from build123d import *

# Parameters (mm, degrees)
BOSS_EXTRUDE1_DEPTH                            = 60
CUT_EXTRUDE1_DEPTH                             = 114.247516529
CBORE_FOR_4_SOCKET_HEAD_CAP_SCREW1_D           = 3.2639
CBORE_FOR_4_SOCKET_HEAD_CAP_SCREW1_CBORE_D     = 5.55752
CBORE_FOR_4_SOCKET_HEAD_CAP_SCREW1_CBORE_DEPTH = 2.8448
CUT_EXTRUDE5_REACH                             = 115.248
CUT_EXTRUDE6_DEPTH                             = 2.84
M3_TAPPED_HOLE1_D                              = 2.5
M3_TAPPED_HOLE1_DEPTH                          = 8.5
M3_TAPPED_HOLE1_TIP                            = 0.751075774
M5_TAPPED_HOLE1_D                              = 4.2
SKETCH11_R                                     = 5
CUT_EXTRUDE2_DEPTH                             = 114.247516529
M4_TAPPED_HOLE1_D                              = 3.3
M4_TAPPED_HOLE1_DEPTH                          = 6
M4_TAPPED_HOLE1_CSINK_D                        = 4.5
M4_TAPPED_HOLE1_CSINK_ANGLE                    = 90
M5_TAPPED_HOLE2_D                              = 4.2
M5_TAPPED_HOLE2_DEPTH                          = 6
M5_TAPPED_HOLE2_CSINK_D                        = 5.05
M5_TAPPED_HOLE2_CSINK_ANGLE                    = 90
SKETCH16_R                                     = 10
CUT_EXTRUDE4_DEPTH                             = 30
M3_TAPPED_HOLE2_AT_2_COUNT                     = 2
M3_TAPPED_HOLE2_AT_2_PITCH                     = 20


with BuildPart() as part:
    # Sketch1 → Boss-Extrude1 (new body)
    with BuildSketch(Plane.XY):
        Polygon((0, 0), (6, 0), (6, 54), (69, 54), (69, 40), (75, 40), (75, 60), (0, 60), align=None)
    extrude(amount=BOSS_EXTRUDE1_DEPTH)

    # Sketch2 → Cut-Extrude1 (cut, through all)
    with BuildSketch(Plane(origin=(0, 60, 0), x_dir=(1, 0, 0), z_dir=(0, 1, 0))):
        with BuildLine():
            Line((40, -18.5), (50, -18.5))
            ThreePointArc((50, -18.5), (61.5, -30), (50, -41.5))
            Line((50, -41.5), (40, -41.5))
            ThreePointArc((40, -41.5), (28.5, -30), (40, -18.5))
        make_face()
    extrude(amount=-CUT_EXTRUDE1_DEPTH, mode=Mode.SUBTRACT)

    # CBORE for #4 Socket Head Cap Screw1 (through all)
    with Locations(Plane(origin=(0, 60, 0), x_dir=(-1, 0, 0), z_dir=(0, 1, 0))):
        with Locations((-24.5, 45.5), (-55.5, 45.5), (-24.5, 14.5), (-55.5, 14.5)):
            CounterBoreHole(CBORE_FOR_4_SOCKET_HEAD_CAP_SCREW1_D / 2, CBORE_FOR_4_SOCKET_HEAD_CAP_SCREW1_CBORE_D / 2, CBORE_FOR_4_SOCKET_HEAD_CAP_SCREW1_CBORE_DEPTH)

    # Sketch24 → Cut-Extrude5 (cut, up to next)
    with BuildSketch(Plane(origin=(0, 60, 0), x_dir=(1, 0, 0), z_dir=(0, 1, 0)), mode=Mode.PRIVATE) as cut_extrude5_sk1:
        with BuildLine():
            Line((24.5, -12.86805), (34.5, -12.86805))
            ThreePointArc((34.5, -12.86805), (36.13195, -14.5), (34.5, -16.13195))
            Line((34.5, -16.13195), (24.5, -16.13195))
            ThreePointArc((24.5, -16.13195), (22.86805, -14.5), (24.5, -12.86805))
        make_face()
    cut_extrude5_tool1 = extrude(cut_extrude5_sk1.sketch, amount=-CUT_EXTRUDE5_REACH, mode=Mode.PRIVATE) & part.part
    # Sketch24 → Cut-Extrude5 (cut, up to next)
    with BuildSketch(Plane(origin=(0, 60, 0), x_dir=(1, 0, 0), z_dir=(0, 1, 0)), mode=Mode.PRIVATE) as cut_extrude5_sk2:
        with BuildLine():
            Line((55.5, -12.86805), (65.5, -12.86805))
            ThreePointArc((65.5, -12.86805), (67.13195, -14.5), (65.5, -16.13195))
            Line((65.5, -16.13195), (55.5, -16.13195))
            ThreePointArc((55.5, -16.13195), (53.86805, -14.5), (55.5, -12.86805))
        make_face()
    cut_extrude5_tool2 = extrude(cut_extrude5_sk2.sketch, amount=-CUT_EXTRUDE5_REACH, mode=Mode.PRIVATE) & part.part
    # Sketch24 → Cut-Extrude5 (cut, up to next)
    with BuildSketch(Plane(origin=(0, 60, 0), x_dir=(1, 0, 0), z_dir=(0, 1, 0)), mode=Mode.PRIVATE) as cut_extrude5_sk3:
        with BuildLine():
            Line((24.5, -43.911016089), (34.5, -43.911016089))
            ThreePointArc((34.5, -43.911016089), (36.13195, -45.542966089), (34.5, -47.174916089))
            Line((34.5, -47.174916089), (24.5, -47.174916089))
            ThreePointArc((24.5, -47.174916089), (22.86805, -45.542966089), (24.5, -43.911016089))
        make_face()
    cut_extrude5_tool3 = extrude(cut_extrude5_sk3.sketch, amount=-CUT_EXTRUDE5_REACH, mode=Mode.PRIVATE) & part.part
    # Sketch24 → Cut-Extrude5 (cut, up to next)
    with BuildSketch(Plane(origin=(0, 60, 0), x_dir=(1, 0, 0), z_dir=(0, 1, 0)), mode=Mode.PRIVATE) as cut_extrude5_sk4:
        with BuildLine():
            Line((55.5, -43.911016089), (65.5, -43.911016089))
            ThreePointArc((65.5, -43.911016089), (67.13195, -45.542966089), (65.5, -47.174916089))
            Line((65.5, -47.174916089), (55.5, -47.174916089))
            ThreePointArc((55.5, -47.174916089), (53.86805, -45.542966089), (55.5, -43.911016089))
        make_face()
    cut_extrude5_tool4 = extrude(cut_extrude5_sk4.sketch, amount=-CUT_EXTRUDE5_REACH, mode=Mode.PRIVATE) & part.part
    add(cut_extrude5_tool1.solids().sort_by_distance((29.5, 60, 14.5))[0], mode=Mode.SUBTRACT)
    add(cut_extrude5_tool2.solids().sort_by_distance((60.5, 60, 14.5))[0], mode=Mode.SUBTRACT)
    add(cut_extrude5_tool3.solids().sort_by_distance((29.5, 60, 45.542966))[0], mode=Mode.SUBTRACT)
    add(cut_extrude5_tool4.solids().sort_by_distance((60.5, 60, 45.542966))[0], mode=Mode.SUBTRACT)

    # Sketch25 → Cut-Extrude6 (cut)
    with BuildSketch(Plane(origin=(0, 60, 0), x_dir=(1, 0, 0), z_dir=(0, 1, 0))):
        with BuildLine():
            Line((24.5, -11.72124), (34.5, -11.72124))
            ThreePointArc((34.5, -11.72124), (37.27876, -14.5), (34.5, -17.27876))
            Line((34.5, -17.27876), (24.5, -17.27876))
            ThreePointArc((24.5, -17.27876), (21.72124, -14.5), (24.5, -11.72124))
        make_face()
        with BuildLine():
            Line((55.499999686, -11.73110797), (65.499999686, -11.73110797))
            ThreePointArc((65.499999686, -11.73110797), (68.278759686, -14.50986797), (65.499999686, -17.28862797))
            Line((65.499999686, -17.28862797), (55.499999686, -17.28862797))
            ThreePointArc((55.499999686, -17.28862797), (52.721239686, -14.50986797), (55.499999686, -11.73110797))
        make_face()
        with BuildLine():
            Line((24.5, -42.822083884), (34.5, -42.822083884))
            ThreePointArc((34.5, -42.822083884), (37.27876, -45.600843884), (34.5, -48.379603884))
            Line((34.5, -48.379603884), (24.5, -48.379603884))
            ThreePointArc((24.5, -48.379603884), (21.72124, -45.600843884), (24.5, -42.822083884))
        make_face()
        with BuildLine():
            Line((55.499999686, -42.831951854), (65.499999686, -42.831951854))
            ThreePointArc((65.499999686, -42.831951854), (68.278759686, -45.610711854), (65.499999686, -48.389471854))
            Line((65.499999686, -48.389471854), (55.499999686, -48.389471854))
            ThreePointArc((55.499999686, -48.389471854), (52.721239686, -45.610711854), (55.499999686, -42.831951854))
        make_face()
    extrude(amount=-CUT_EXTRUDE6_DEPTH, mode=Mode.SUBTRACT)

    # M3 Tapped Hole1
    with Locations(Plane(origin=(0, 60, 0), x_dir=(-1, 0, 0), z_dir=(0, 1, 0))):
        with Locations((-12, 55), (-72, 55), (-12, 5), (-72, 5)):
            Hole(M3_TAPPED_HOLE1_D / 2, depth=M3_TAPPED_HOLE1_DEPTH)
            with Locations((0, 0, -(M3_TAPPED_HOLE1_DEPTH + M3_TAPPED_HOLE1_TIP / 2))):  # 118° drill point
                Cone(0, M3_TAPPED_HOLE1_D / 2, M3_TAPPED_HOLE1_TIP, mode=Mode.SUBTRACT)

    # M5 Tapped Hole1 (through all)
    with Locations(Plane(origin=(0, 60, 0), x_dir=(-1, 0, 0), z_dir=(0, 1, 0))):
        with Locations((-44, 12), (-44, 48)):
            Hole(M5_TAPPED_HOLE1_D / 2)

    # Sketch11 → Cut-Extrude2 (cut, through all)
    with BuildSketch(Plane(origin=(0, 60, 0), x_dir=(1, 0, 0), z_dir=(0, 1, 0))):
        with Locations(Location((12, -30, 0), (0, 0, 270))):
            Circle(SKETCH11_R)
    extrude(amount=-CUT_EXTRUDE2_DEPTH, mode=Mode.SUBTRACT)

    # M4 Tapped Hole1
    with Locations(Plane.ZY):
        with Locations((11, 46), (11, 16), (49, 46), (49, 16)):
            CounterSinkHole(M4_TAPPED_HOLE1_D / 2, M4_TAPPED_HOLE1_CSINK_D / 2, depth=M4_TAPPED_HOLE1_DEPTH, counter_sink_angle=M4_TAPPED_HOLE1_CSINK_ANGLE)

    # M5 Tapped Hole2
    with Locations(Plane(origin=(75, 0, 0), x_dir=(0, 0, -1), z_dir=(1, 0, 0))):
        with Locations((-30, 50)):
            CounterSinkHole(M5_TAPPED_HOLE2_D / 2, M5_TAPPED_HOLE2_CSINK_D / 2, depth=M5_TAPPED_HOLE2_DEPTH, counter_sink_angle=M5_TAPPED_HOLE2_CSINK_ANGLE)

    # Sketch16 → Cut-Extrude4 (cut)
    with BuildSketch(Plane.XZ):
        with Locations((12, 30)):
            Circle(SKETCH16_R)
    extrude(amount=-CUT_EXTRUDE4_DEPTH, mode=Mode.SUBTRACT)

    # Sketch29 → M3 Tapped Hole2 (revolve, cut)
    with BuildSketch(Plane(origin=(12, 54, 40), x_dir=(0, 0, -1), z_dir=(1, 0, 0))):
        Polygon((0, 0), (0, 6), (1.525, 6), (1.25, 5.725), (1.25, 0.275), (1.525, 0), align=None)
    m3_tapped_hole2 = revolve(axis=Axis((12, 47.65, 40), (0, 1, 0)), mode=Mode.SUBTRACT)

    # M3 Tapped Hole2 at 2: M3 Tapped Hole2 ×2
    with Locations(*[(0, 0, -i * M3_TAPPED_HOLE2_AT_2_PITCH) for i in range(1, M3_TAPPED_HOLE2_AT_2_COUNT)]):
        add(m3_tapped_hole2, mode=Mode.SUBTRACT)


solid = part.part
Here's how the part is built. I have some questions about the finished solid (model axes, mm). A direction names the side the tool comes from. Round coordinates to 2 decimals unless told otherwise and drop trailing zeros. Write each loop counter-clockwise with the first axis right and the second up, starting at its lowest first coordinate (ties: lowest second). Pieces come first, ordered by that corner, then holes.
1. Suppose I cut it at D-D (x = 19). List the corners of the cut face in (y, z) for me, and give its area (3 significant figures).
2. For faces 4 (the flat face through (61, 59, 11.731)), 5 (the flat face through (72, 40, 30)), 6 (the cylindrical face through (36.13, 55.6, 14.46)), 7 (the flat face through (0, 30, 30)), which set-ups out of +Z, -Z, +X, -X, +Y, -Y let a thin tool reach every point of the face, with its end or its side?
3. I need wall thicknesses on L1, parallel to X at y = 47.5, z = 26.5; L2, parallel to Z at x = 55.5, y = 59.4; L3, parallel to Y at x = 57.5, z = 55.5. Which ranges of each line are inside material? Lowest first, please.
4. Will these pins go through, and if not, where does the flat tip stop? pin 1 Ø1 at (y, z) = (17, 40) entering from +X; pin 2 Ø1.2 at (x, z) = (4, 33) entering from -Y; pin 3 Ø3 at (x, z) = (12, 40) entering from +Y (3 decimals).
5. Suppose I cut it at B-B (z = 40). List the corners of the cut face in (x, y) for me (3 decimals), and give its area (3 significant figures).
6. Suppose I cut it at C-C (y = 7). List the corners of the cut face in (x, z) for me, and give its area (3 significant figures).
7. Suppose I cut it at A-A (x = 64). List the corners of the cut face in (y, z) for me.
8. If we mould it in two halves opening along Y, with no side actions, what happens to faces 1 (the cylindrical face through (10.946, 56.962, 19.328)), 2 (the flat face through (4, 30, 30)), 3 (the cylindrical face through (3.338, 15.368, 9.476))? For each: released by +Y, released by -Y, zero draft, split by the parting line, or undercut.
Answer sheet:
1. outline: (54, 0) - (60, 0) - (60, 60) - (54, 60) - close
1. area: 360 mm2
2. face 4: +Y
2. face 5: +Z, -Z, +X, -Y
2. face 6: +Y, -Y
2. face 7: +Z, -Z, -X, +Y, -Y
3. L1: x = 0 to 6, 69 to 75
3. L2: z = 0 to 11.72, 17.29 to 19.9, 40.1 to 42.72, 48.39 to 60
3. L3: y = 54 to 60
4. pin 1: stops at x = 6
4. pin 2: stops at y = 30
4. pin 3: stops at y = 59.975
5. outline: (0, 0) - (6, 0) - (6, 54) - (10.475, 54) - (10.75, 54.275) - (10.75, 59.725) - (10.475, 60) - (0, 60) - close; (13.25, 54.275) - (13.525, 54) - (34.321, 54) - (34.321, 60) - (13.525, 60) - (13.25, 59.725) - close; (55.679, 54) - (69, 54) - (69, 40) - (75, 40) - (75, 60) - (55.679, 60) - close
5. area: 715 mm2
6. outline: (0, 0) - (6, 0) - (6, 22) arc R10 cw to (6, 38) - (6, 60) - (0, 60) - close
6. area: 315 mm2
7. outline: (54, 0) - (60, 0) - (60, 11.73) - (57.16, 11.73) - (57.16, 12.87) - (54, 12.87) - close; (54, 16.13) - (57.16, 16.13) - (57.16, 17.29) - (60, 17.29) - (60, 42.83) - (57.16, 42.83) - (57.16, 43.91) - (54, 43.91) - close; (54, 47.17) - (57.16, 47.17) - (57.16, 48.39) - (60, 48.39) - (60, 60) - (54, 60) - close
8. face 1: zero draft
8. face 2: released by -Y
8. face 3: undercut
